Work out the finished part from the listing and answer in its coordinate system (mm). A direction names the side the tool comes from. Round coordinates to 2 decimals unless told otherwise and drop trailing zeros. Order: outer loops, then holes, each group sorted by start corner. A loop starts at its lowest first (then second) coordinate and runs counter-clockwise, first axis right, second up. Notation, with made-up numbers: (13, 80.5) - (28, 80.5) arc R36 ccw to (28, 114.5) - close; hole circle Ø7 at (12, 42.5). An arc over 180 degrees is marked (long way). Use CSV: the item, a comma, the result in double quotes.
Autodesk Fusion 360 part; units mm, degrees
sketch "Sketch1" plane through (0, 0, 0) normal (1, 0, 0) x (0, 1, 0)
  line L0 (17.5, -20) -> (-17.5, -20)
  line L1 (-17.5, -20) -> (-17.5, 20)
  line L2 (-17.5, 20) -> (17.5, 20)
  line L3 (17.5, 20) -> (17.5, -20)
  line L4 (17.5, -20) -> (-17.5, 20) construction
  line L5 (-17.5, -20) -> (17.5, 20) construction
  line L6 (0.5, 11.5) -> (-0.5, 11.5)
  line L7 (-4.5, 7.5) -> (-4.5, -7.5)
  line L8 (-0.5, -11.5) -> (0.5, -11.5)
  line L9 (4.5, -7.5) -> (4.5, 7.5)
  line L10 (4.5, 11.5) -> (-4.5, -11.5) construction
  line L11 (-4.5, 11.5) -> (4.5, -11.5) construction
  arc A0 (-0.5, 11.5) -> (-4.5, 7.5) centre (-0.5, 7.5) ccw
  arc A1 (4.5, 7.5) -> (0.5, 11.5) centre (0.5, 7.5) ccw
  arc A2 (-4.5, -7.5) -> (-0.5, -11.5) centre (-0.5, -7.5) ccw
  arc A3 (0.5, -11.5) -> (4.5, -7.5) centre (0.5, -7.5) ccw
  dimension "d1" = 35
  dimension "d2" = 40
  dimension "d3" = 9
  dimension "d4" = 23
  dimension "d5" = 4
  dimension "d6" = 4
  dimension "d7" = 4
  dimension "d8" = 4
extrude "Extrude1" add sketch "Sketch1" along normal blind 4
sketch "Sketch2" plane through (0, 0, -20) normal (0, 0, -1) x (1, 0, 0)
  line L0 (0, 17.5) -> (0, -17.5)
  line L1 (0, -17.5) -> (4, -17.5)
  line L2 (4, -17.5) -> (4, 17.5)
  line L3 (4, 17.5) -> (0, 17.5)
  line L4 (4, -17.5) -> (40, -17.5)
  line L5 (40, -17.5) -> (40, 17.5)
  line L6 (40, 17.5) -> (4, 17.5)
  line L7 (4, -17.5) -> (4, 17.5)
  line L8 (12.5, 4.5) -> (27.5, 4.5)
  line L9 (31.5, 0.5) -> (31.5, -0.5)
  line L10 (27.5, -4.5) -> (12.5, -4.5)
  line L11 (8.5, -0.5) -> (8.5, 0.5)
  line L12 (8.5, 4.5) -> (31.5, -4.5) construction
  line L13 (31.5, 4.5) -> (8.5, -4.5) construction
  arc A0 (27.5, -4.5) -> (31.5, -0.5) centre (27.5, -0.5) ccw
  arc A1 (8.5, -0.5) -> (12.5, -4.5) centre (12.5, -0.5) ccw
  arc A2 (12.5, 4.5) -> (8.5, 0.5) centre (12.5, 0.5) ccw
  arc A3 (31.5, 0.5) -> (27.5, 4.5) centre (27.5, 0.5) ccw
  point P0 (20, -17.5)
  point P1 (20, 0)
  point P2 (20, 0)
  dimension "d11" = 40
  dimension "d13" = 17.5
  dimension "d14" = 20
  dimension "d15" = 23
  dimension "d16" = 9
  dimension "d17" = 4
  dimension "d18" = 4
  dimension "d19" = 4
  dimension "d20" = 4
extrude "Extrude2" add sketch "Sketch2" against normal blind 4 contours L2 L4 L5 L6 L7
sketch "Sketch3" plane through (0, 17.5, 0) normal (0, 1, 0) x (-1, 0, 0)
  line L0 (0, -20) -> (0, 20)
  line L1 (0, 20) -> (-4, 20)
  line L2 (-4, 20) -> (-4, -16)
  line L3 (-4, -16) -> (-40, -16)
  line L4 (-40, -16) -> (-40, -20)
  line L5 (-40, -20) -> (0, -20)
  line L6 (-4, 20) -> (-5.2, 20)
  line L7 (-5.2, -16) -> (-4, -16)
  line L8 (-4, -16) -> (-4, 20)
  line L9 (-40, -16) -> (-5.2, -16)
  line L10 (-5.2, -16) -> (-5.2, -14.8)
  line L11 (-35, -14.8) -> (-40, -14.8)
  line L12 (-40, -14.8) -> (-40, -16)
  line L13 (-35, -14.8) -> (-5.2, 15)
  line L14 (-35, -14.8) -> (6.8148, -14.8) construction
  line L15 (-5.2, 20) -> (-5.2, 15)
  line L16 (-5.2, -14.8) -> (-5.2, -16)
  dimension "d23" = 1.2
  dimension "d24" = 1.2
  dimension "d25" = 45
  dimension "d26" = 5
extrude "Extrude3" add sketch "Sketch3" against normal blind 4 contours L2 L3 L6 L7 L8 L9 L11 L12 L13 L15
sketch "Sketch4" plane through (0, -17.5, 0) normal (0, -1, 0) x (1, 0, 0)
  line L0 (0, 20) -> (0, -20)
  line L1 (0, -20) -> (40, -20)
  line L2 (40, -20) -> (40, -16)
  line L3 (40, -16) -> (4, -16)
  line L4 (4, -16) -> (4, 20)
  line L5 (4, 20) -> (0, 20)
  line L6 (4, 20) -> (5.2, 20)
  line L7 (5.2, 20) -> (5.2, 15)
  line L8 (5.2, 15) -> (35, -14.8)
  line L9 (35, -14.8) -> (40, -14.8)
  line L10 (40, -14.8) -> (40, -16)
  dimension "d29" = 1.2
extrude "Extrude4" add sketch "Sketch4" against normal blind 4 contours L3 L4 L6 L7 L8 L9 L10
(1) For faces 4 (the flat face through (2, 0, -11.5)), 5 (the flat face through (14, -13.5, -6)), 6 (the cylindrical face through (30.297, 3.359, -18.028)), determine the directions among +Z, -Z, +X, -X, +Y, -Y from which every point of the face is accessible in a straight line to the end or side of a thin tool.
Findings below:
face 4,"+X, -X"
face 5,"+Z, +X"
face 6,"+Z, -Z"
(2) Find section A-A (z = 3.5). Determine the outline of the cut face in (x, y).
Findings below:
outline,"(0, -17.5) - (16.7, -17.5) - (16.7, -13.5) - (4, -13.5) - (4, -4.5) - (0, -4.5) - close; (0, 4.5) - (4, 4.5) - (4, 13.5) - (16.7, 13.5) - (16.7, 17.5) - (0, 17.5) - close"
(3) Find the intervals of material crossed by L1, parallel to Y at x = 10.5, z = 6.5; L2, parallel to X at y = 4.5, z = -11.5; L3, parallel to Z at x = 30.5, y = -13, in increasing order. Write a range as from..to.
Findings below:
L1,"y = -17.5..-13.5, 13.5..17.5"
L2,"x = 0..4"
L3,"z = -20..-16"
(4) Find section B-B (x = 19). Determine the outline of the cut face in (y, z).
Findings below:
outline,"(-17.5, -20) - (-4.5, -20) - (-4.5, -16) - (-13.5, -16) - (-13.5, 1.2) - (-17.5, 1.2) - close; (4.5, -20) - (17.5, -20) - (17.5, 1.2) - (13.5, 1.2) - (13.5, -16) - (4.5, -16) - close"
(5) Each of these flat-tipped pins is pushed along its axis until it touches: pin 1 (3 mm diameter, centred on y = 8, z = -2, fed in from +X); pin 2 (13.5 mm diameter, centred on x = 15, y = 1, fed in from +Z); pin 3 (2 mm diameter, centred on y = 14.5, z = 17.5, fed in from +X); pin 4 (1.1 mm diameter, centred on y = 0, z = -17.5, fed in from -X). Where does it stop, or does it pass through?
Findings below:
pin 1,"stops at x = 4"
pin 2,"stops at z = -16"
pin 3,"stops at x = 5.2"
pin 4,"stops at x = 0"
(6) Find section C-C (y = -8). Determine the outline of the cut face in (x, z).
Findings below:
outline,"(0, -20) - (40, -20) - (40, -16) - (4, -16) - (4, 20) - (0, 20) - close"
(7) The mould has two halves that part along X. Classify faces 1 (the flat face through (20, -8, -20)), 2 (the flat face through (5.2, -16, 18)), 3 (the cylindrical face through (30.359, -3.297, -18.028)): released by +X, released by -X, zero draft, split by the parting line, or undercut.
Findings below:
face 1,"zero draft"
face 2,"released by +X"
face 3,"undercut"
(8) Find section D-D (z = -12.5). Determine the outline of the cut face in (x, y), and give its area (3 significant figures).
Findings below:
outline,"(0, -17.5) - (32.7, -17.5) - (32.7, -13.5) - (4, -13.5) - (4, 13.5) - (32.7, 13.5) - (32.7, 17.5) - (0, 17.5) - close"
area,"370 mm²"
